```python
from build123d import *

# Parameters (mm, degrees)
SALIENTE_EXTRUIR1_DEPTH = 3
CORTAR_EXTRUIR1_DEPTH   = 10


with BuildPart() as part:
    # Croquis1 → Saliente-Extruir1 (new body)
    with BuildSketch(Plane(origin=(0, 0, 0), x_dir=(0, 0, -1), z_dir=(1, 0, 0))):
        Polygon((-40, 0), (40, 0), (40, -20), (43, -20), (43, -35), (40, -35), (40, -55), (-40, -55), (-40, -35), (-43, -35), (-43, -20), (-40, -20), align=None)
    extrude(amount=SALIENTE_EXTRUIR1_DEPTH)

    # Croquis2 → Cortar-Extruir1 (cut)
    with BuildSketch(Plane.ZY):
        Polygon((-40, -8.5), (-32, -8.5), (-32, -6.5), (-29, -6.5), (-29, -8.5), (-25, -8.5), (-25, -11.5), (-29, -11.5), (-29, -13.5), (-32, -13.5), (-32, -11.5), (-40, -11.5), align=None)
        Polygon((29, -11.5), (25, -11.5), (25, -8.5), (29, -8.5), (29, -6.5), (32, -6.5), (32, -8.5), (40, -8.5), (40, -11.5), (32, -11.5), (32, -13.5), (29, -13.5), align=None)
        Polygon((-12, 0), (-12, -8), (-10, -8), (-10, -11), (-12, -11.013841386), (-12, -15), (-15, -15), (-15, -11.034603466), (-17, -11.048444852), (-17, -8), (-15, -8), (-15, 0), align=None)
        Polygon((15, -11.034603466), (15, -15), (12, -15), (12, -11.013841386), (10, -11), (10, -8), (12, -8), (12, 0), (15, 0), (15, -8), (17, -8), (17, -11.048444852), align=None)
        Polygon((40, -46.5), (32, -46.5), (32, -48.5), (29, -48.5), (29, -46.5), (25, -46.5), (25, -43.5), (29, -43.5), (29, -41.5), (32, -41.5), (32, -43.5), (40, -43.5), align=None)
        Polygon((-29, -43.5), (-25, -43.5), (-25, -46.5), (-29, -46.5), (-29, -48.5), (-32, -48.5), (-32, -46.5), (-40, -46.5), (-40, -43.5), (-32, -43.5), (-32, -41.5), (-29, -41.5), align=None)
    extrude(amount=-CORTAR_EXTRUIR1_DEPTH, mode=Mode.SUBTRACT)


solid = part.part
```
Read the model definition and answer for the solid it produces. Units are mm, in the model's axes. A direction names the side the tool comes from. Coordinates: 2 decimals unless noted, no trailing zeros. Loops run counter-clockwise (first coordinate to the right, second up) from the corner with the lowest first, then second, coordinate; pieces in that order, holes last. Notation, with made-up numbers: (39, 17) -> (46, 17) arc R21 cw to (46, 38) -> close; hole circle Ø1 at (-21.75, 27). An arc over 180 degrees is marked (long way). Return JSON: item names as keys, results as strings.
Item 1: Find section A-A (y = -12.5). Determine the outline of the cut face in (x, z), plus the area to 3 significant figures.
Answers:
{"outline": "(0, -40) -> (3, -40) -> (3, -32) -> (0, -32) -> close; (0, -29) -> (3, -29) -> (3, -15) -> (0, -15) -> close; (0, -12) -> (3, -12) -> (3, 12) -> (0, 12) -> close; (0, 15) -> (3, 15) -> (3, 29) -> (0, 29) -> close; (0, 32) -> (3, 32) -> (3, 40) -> (0, 40) -> close", "area": "204 mm2"}
Item 2: Find the intervals of material crossed by probe 1 along Y at (x, z) = (0.3, 34.5); probe 2 along Z at (x, y) = (1.2, -42); probe 3 along Z at (x, y) = (1.1, -6), in increasing order.
Answers:
{"probe 1": "y = -55 to -46.5, -43.5 to -11.5, -8.5 to 0", "probe 2": "z = -40 to -32, -29 to 29, 32 to 40", "probe 3": "z = -40 to -15, -12 to 12, 15 to 40"}
Item 3: Find section B-B (y = -42.5). Determine the outline of the cut face in (x, z), plus the area to 3 significant figures.
Answers:
{"outline": "(0, -40) -> (3, -40) -> (3, -32) -> (0, -32) -> close; (0, -29) -> (3, -29) -> (3, 29) -> (0, 29) -> close; (0, 32) -> (3, 32) -> (3, 40) -> (0, 40) -> close", "area": "222 mm2"}
Item 4: For a pull along Z with two mould halves and no side action, classify faces 4 (the flat face through (1, -51, -40)), 5 (the flat face through (1, -48, -32)), 6 (the flat face through (1, -35, -42)), 7 (the flat face through (1, -13.5, -30)) as +Z half, -Z half, draft (parallel to the pull), parting line (faces both ways), or undercut.
Answers:
{"face 4": "-Z half", "face 5": "undercut", "face 6": "draft", "face 7": "undercut"}
Item 5: Flat-ended cylindrical pins translate along their axes: P1, Ø0.6, axis at x = 1, y = -7.5, coming from the +Z side; P2, Ø1.5, axis at x = 2, z = 14, coming from the +Y side. Find the tip coordinate at first contact, or state that the pin passes through.
Answers:
{"P1": "stops at z = 40", "P2": "stops at y = -15"}
Item 6: Find section C-C (z = -14). Determine the outline of the cut face in (x, y).
Answers:
{"outline": "(0, -55) -> (3, -55) -> (3, -15) -> (0, -15) -> close"}
Item 7: Find section D-D (y = -36). Determine the outline of the cut face in (x, z), plus the area to 3 significant figures.
Answers:
{"outline": "(0, -40) -> (3, -40) -> (3, 40) -> (0, 40) -> close", "area": "240 mm2"}
Item 8: For faces 1 (the flat face through (1, -45, 25)), 2 (the flat face through (1, -51, 40)), 3 (the flat face through (1, -10, 17)), determine the directions among +Z, -Z, +X, -X, +Y, -Y from which every point of the face is accessible in a straight line to the end or side of a thin tool.
Answers:
{"face 1": "+Z, +X, -X", "face 2": "+Z, +X, -X, -Y", "face 3": "+X, -X"}
